The listing builds one solid part. Answer for the finished solid, in the listing's coordinates (mm). Coordinates: 2 decimals unless noted, no trailing zeros. Order: outer loops, then holes, each group sorted by start corner. A loop starts at its lowest first (then second) coordinate and runs counter-clockwise, first axis right, second up. Notation, with made-up numbers: (-35, 41.5) -> (-29, 41.5) arc R18 ccw to (-29, 46.5) -> close; hole circle Ø9 at (-20.75, -32.5). An arc over 180 degrees is marked (long way). Write item = value, one per line.
from build123d import *

# Parameters (mm, degrees)
SKETCH1_W           = 250
SKETCH1_H           = 300
BOSS_EXTRUDE1_DEPTH = 100
SKETCH2_W           = 15
SKETCH2_H           = 15
BOSS_EXTRUDE2_DEPTH = 7.5
FILLET1_R           = 7.5


with BuildPart() as part:
    # Sketch1 → Boss-Extrude1 (new body)
    with BuildSketch(Plane.XY):
        Rectangle(SKETCH1_W, SKETCH1_H)
    extrude(amount=BOSS_EXTRUDE1_DEPTH)

    # Sketch2 → Boss-Extrude2 (add)
    with BuildSketch(Plane(origin=(0, 0, 0), x_dir=(-1, 0, 0), z_dir=(0, 0, -1))):
        with Locations((0, 100)):
            Rectangle(SKETCH2_W, SKETCH2_H)
        with Locations((0, -100)):
            Rectangle(SKETCH2_W, SKETCH2_H)
    extrude(amount=BOSS_EXTRUDE2_DEPTH)

    # Fillet1
    fillet1_edges = [part.edges().sort_by_distance(p)[0] for p in [
        (0, 107.5, -7.5),
        (0, 92.5, -7.5),
        (0, -107.5, -7.5),
        (0, -92.5, -7.5),
    ]]
    fillet(fillet1_edges, radius=FILLET1_R - 0.0001)  # a hair under: the kernel refuses the full size


solid = part.part
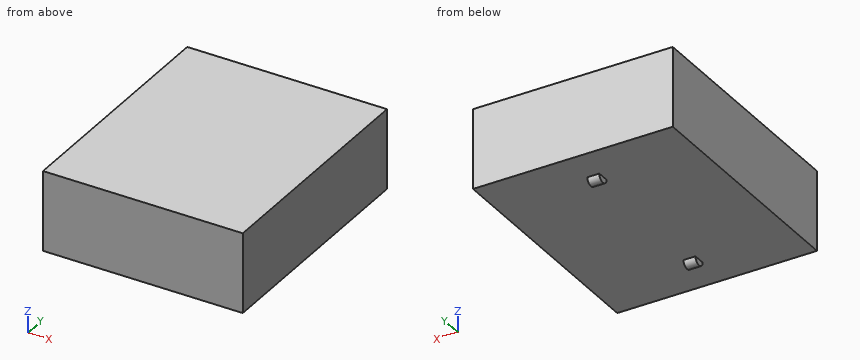
Q1. Section A-A, the plane y = 27 is taken. Give the vertices of the cut face in (x, z).
The answers:
outline = (-125, 0) -> (125, 0) -> (125, 100) -> (-125, 100) -> close
Q2. Each of these flat-tipped pins is pushed along its axis until it touches: pin 1 Ø2 at (y, z) = (-97, -4) entering from +X; pin 2 Ø8.5 at (y, z) = (-99, -5.5) entering from -X; pin 3 Ø3 at (x, y) = (-48.5, 82.5) entering from -Z. Where does it stop, or does it pass through?
The answers:
pin_1 = 7.5
pin_2 = -7.5
pin_3 = 0
Q3. Find the intervals of material crossed by line 1 along Z through (x, y) = (-105.5, -126), in increasing order.
The answers:
line_1 = 0 to 100
Q4. Section B-B, the plane x = -83.5 is taken. Give the vertices of the cut face in (y, z).
The answers:
outline = (-150, 0) -> (150, 0) -> (150, 100) -> (-150, 100) -> close
